```python
from build123d import *

# Parameters (mm, degrees)
CUT_EXTRUDE1_DEPTH  = 153.548755526
CIRPATTERN1_COUNT   = 4
SKETCH6_W           = 0.3175
SKETCH6_H           = 19.05
CUT_EXTRUDE3_DEPTH  = 154.364331947
BOSS_EXTRUDE1_START = 6.19125
SKETCH7_R           = 4.6355
BOSS_EXTRUDE1_DEPTH = 14.76375
FILLET1_R           = 0.9525


with BuildPart() as part:
    # Sketch2 → Revolve1 (revolve)
    with BuildSketch(Plane(origin=(0, 0, 0), x_dir=(0, 0, -1), z_dir=(1, 0, 0)), mode=Mode.PRIVATE) as revolve1_sk:
        Polygon((-133.35, -4.7625), (152.4, -4.7625), (152.4, 0), (-152.4, 0), (-152.4, -4.7625), align=None)
    revolve(revolve1_sk.sketch.rotate(Axis((0, 0, 152.4), (0, 0, -1)), 270), axis=Axis((0, 0, 152.4), (0, 0, -1)))

    # Sketch3 → Cut-Extrude1 (cut, symmetric)
    with BuildSketch(Plane(origin=(0, 0, 0), x_dir=(0, 0, -1), z_dir=(1, 0, 0))):
        Polygon((-152.4, -0.00254), (-133.35, -4.7625), (-152.4, -4.7625), align=None)
    cut_extrude1 = extrude(amount=CUT_EXTRUDE1_DEPTH, both=True, mode=Mode.SUBTRACT)

    # CirPattern1: Cut-Extrude1 ×4 about axis
    cirpattern1_axis = Axis((0, 0, 0), (0, 0, 1))
    for i in range(1, CIRPATTERN1_COUNT):
        add(cut_extrude1.rotate(cirpattern1_axis, i * 360 / CIRPATTERN1_COUNT), mode=Mode.SUBTRACT)

    # Sketch5 → Revolve2 (revolve)
    with BuildSketch(Plane(origin=(0, 0, 0), x_dir=(0, 0, -1), z_dir=(1, 0, 0)), mode=Mode.PRIVATE) as revolve2_sk:
        with BuildLine():
            Line((148.828125, 0), (152.4, 0))
            Line((152.4, 0), (152.4, 8.105021576))
            ThreePointArc((152.4, 8.105021576), (152.243002117, 8.716680214), (151.810824742, 9.177111904))
            ThreePointArc((151.810824742, 9.177111904), (150.6140625, 9.525), (149.417300258, 9.177111904))
            ThreePointArc((149.417300258, 9.177111904), (148.985122883, 8.716680214), (148.828125, 8.105021576))
            Line((148.828125, 8.105021576), (148.828125, 0))
        make_face()
    revolve(revolve2_sk.sketch.rotate(Axis((0, 0, -152.4), (0, 0, 1)), 90), axis=Axis((0, 0, -152.4), (0, 0, 1)))

    # Sketch6 → Cut-Extrude3 (cut, through all)
    with BuildSketch(Plane(origin=(4.7625, 0, 0), x_dir=(0, 0, -1), z_dir=(1, 0, 0))):
        with Locations((140.414375, 0)):
            Rectangle(SKETCH6_W, SKETCH6_H)
        with Locations((142.478125, 0)):
            Rectangle(SKETCH6_W, SKETCH6_H)
        with Locations((141.44625, 0)):
            Rectangle(SKETCH6_W, SKETCH6_H)
        with Locations((139.3825, 0)):
            Rectangle(SKETCH6_W, SKETCH6_H)
        with Locations((138.350625, 0)):
            Rectangle(SKETCH6_W, SKETCH6_H)
        with Locations((137.31875, 0)):
            Rectangle(SKETCH6_W, SKETCH6_H)
        with Locations((136.286875, 0)):
            Rectangle(SKETCH6_W, SKETCH6_H)
        with Locations((135.255, 0)):
            Rectangle(SKETCH6_W, SKETCH6_H)
        with Locations((134.223125, 0)):
            Rectangle(SKETCH6_W, SKETCH6_H)
        with Locations((133.19125, 0)):
            Rectangle(SKETCH6_W, SKETCH6_H)
        with Locations((132.159375, 0)):
            Rectangle(SKETCH6_W, SKETCH6_H)
        with Locations((131.1275, 0)):
            Rectangle(SKETCH6_W, SKETCH6_H)
        with Locations((130.095625, 0)):
            Rectangle(SKETCH6_W, SKETCH6_H)
        with Locations((129.06375, 0)):
            Rectangle(SKETCH6_W, SKETCH6_H)
        with Locations((128.031875, 0)):
            Rectangle(SKETCH6_W, SKETCH6_H)
    extrude(amount=-CUT_EXTRUDE3_DEPTH, mode=Mode.SUBTRACT)


with BuildPart() as cut_extrude3_piece_1:
    # of the separate pieces the step leaves, piece 1, a body of its own (cut_extrude3_pieces)
    add(part.part.solids().sort_by_distance((4.7625, 0, -127.873125))[0])



with BuildPart() as cut_extrude3_piece_2:
    # of the separate pieces the step leaves, piece 2, a body of its own (cut_extrude3_pieces)
    add(part.part.solids().sort_by_distance((-8.105021576, 0, -152.4))[0])


with BuildPart() as cut_extrude3_piece_3:
    # of the separate pieces the step leaves, piece 3, a body of its own (cut_extrude3_pieces)
    add(part.part.solids().sort_by_distance((4.7625, 0, -142.319375))[0])


with BuildPart() as cut_extrude3_piece_4:
    # of the separate pieces the step leaves, piece 4, a body of its own (cut_extrude3_pieces)
    add(part.part.solids().sort_by_distance((4.7625, 0, -141.2875))[0])


with BuildPart() as cut_extrude3_piece_5:
    # of the separate pieces the step leaves, piece 5, a body of its own (cut_extrude3_pieces)
    add(part.part.solids().sort_by_distance((4.7625, 0, -138.191875))[0])


with BuildPart() as cut_extrude3_piece_6:
    # of the separate pieces the step leaves, piece 6, a body of its own (cut_extrude3_pieces)
    add(part.part.solids().sort_by_distance((4.7625, 0, -137.16))[0])


with BuildPart() as cut_extrude3_piece_7:
    # of the separate pieces the step leaves, piece 7, a body of its own (cut_extrude3_pieces)
    add(part.part.solids().sort_by_distance((4.7625, 0, -136.128125))[0])


with BuildPart() as cut_extrude3_piece_8:
    # of the separate pieces the step leaves, piece 8, a body of its own (cut_extrude3_pieces)
    add(part.part.solids().sort_by_distance((4.7625, 0, -134.064375))[0])


with BuildPart() as cut_extrude3_piece_9:
    # of the separate pieces the step leaves, piece 9, a body of its own (cut_extrude3_pieces)
    add(part.part.solids().sort_by_distance((4.7625, 0, -133.0325))[0])


with BuildPart() as cut_extrude3_piece_10:
    # of the separate pieces the step leaves, piece 10, a body of its own (cut_extrude3_pieces)
    add(part.part.solids().sort_by_distance((4.7625, 0, -132.000625))[0])


with BuildPart() as cut_extrude3_piece_11:
    # of the separate pieces the step leaves, piece 11, a body of its own (cut_extrude3_pieces)
    add(part.part.solids().sort_by_distance((4.7625, 0, -130.96875))[0])


with BuildPart() as cut_extrude3_piece_12:
    # of the separate pieces the step leaves, piece 12, a body of its own (cut_extrude3_pieces)
    add(part.part.solids().sort_by_distance((4.7625, 0, -129.936875))[0])


with BuildPart() as cut_extrude3_piece_13:
    # of the separate pieces the step leaves, piece 13, a body of its own (cut_extrude3_pieces)
    add(part.part.solids().sort_by_distance((4.7625, 0, -128.905))[0])


with BuildPart() as cut_extrude3_piece_14:
    # of the separate pieces the step leaves, piece 14, a body of its own (cut_extrude3_pieces)
    add(part.part.solids().sort_by_distance((4.7625, 0, -140.255625))[0])


with BuildPart() as cut_extrude3_piece_15:
    # of the separate pieces the step leaves, piece 15, a body of its own (cut_extrude3_pieces)
    add(part.part.solids().sort_by_distance((4.7625, 0, -139.22375))[0])


with BuildPart() as cut_extrude3_piece_16:
    # of the separate pieces the step leaves, piece 16, a body of its own (cut_extrude3_pieces)
    add(part.part.solids().sort_by_distance((4.7625, 0, -135.09625))[0])


with BuildPart() as cut_extrude3_piece_1_1:
    add(cut_extrude3_piece_1.part)

    add(cut_extrude3_piece_2.part)  # Boss-Extrude1 merges Cut-Extrude3 piece 2

    add(cut_extrude3_piece_3.part)  # Boss-Extrude1 merges Cut-Extrude3 piece 3

    add(cut_extrude3_piece_4.part)  # Boss-Extrude1 merges Cut-Extrude3 piece 4

    add(cut_extrude3_piece_5.part)  # Boss-Extrude1 merges Cut-Extrude3 piece 5

    add(cut_extrude3_piece_6.part)  # Boss-Extrude1 merges Cut-Extrude3 piece 6

    add(cut_extrude3_piece_7.part)  # Boss-Extrude1 merges Cut-Extrude3 piece 7

    add(cut_extrude3_piece_8.part)  # Boss-Extrude1 merges Cut-Extrude3 piece 8

    add(cut_extrude3_piece_9.part)  # Boss-Extrude1 merges Cut-Extrude3 piece 9

    add(cut_extrude3_piece_10.part)  # Boss-Extrude1 merges Cut-Extrude3 piece 10

    add(cut_extrude3_piece_11.part)  # Boss-Extrude1 merges Cut-Extrude3 piece 11

    add(cut_extrude3_piece_12.part)  # Boss-Extrude1 merges Cut-Extrude3 piece 12

    add(cut_extrude3_piece_13.part)  # Boss-Extrude1 merges Cut-Extrude3 piece 13

    add(cut_extrude3_piece_14.part)  # Boss-Extrude1 merges Cut-Extrude3 piece 14

    add(cut_extrude3_piece_15.part)  # Boss-Extrude1 merges Cut-Extrude3 piece 15

    add(cut_extrude3_piece_16.part)  # Boss-Extrude1 merges Cut-Extrude3 piece 16
    # Sketch7 → Boss-Extrude1 (add)
    with BuildSketch(Plane.XY.offset(-148.828125).offset(BOSS_EXTRUDE1_START)):
        with Locations(Location((0, 0, 0), (0, 0, 180))):
            Circle(SKETCH7_R)
    extrude(amount=BOSS_EXTRUDE1_DEPTH)

    # Fillet1
    fillet1_edges = [cut_extrude3_piece_1_1.edges().sort_by_distance(p)[0] for p in [
        (-4.7625, 0, -148.828125),
    ]]
    fillet(fillet1_edges, radius=FILLET1_R)


solid = cut_extrude3_piece_1_1.part
```
The listing builds one solid part. Answer for the finished solid, in the listing's coordinates (mm). A direction names the side the tool comes from. Give positions to 0.01 mm unless a question says otherwise; leave off trailing zeros. Order: outer loops, then holes, each group sorted by start corner. A loop starts at its lowest first (then second) coordinate and runs counter-clockwise, first axis right, second up. Notation, with made-up numbers: M 84.25,-3.5 L 108.25,-3.5 A29 cw 108.25,31.5 Z; hole C -25.5,-9 d8. An arc over 180 degrees is marked long. Put each result on its own line as item: value. Start each with the question number.
Item 1: Which of the six approach directions +Z, -Z, +X, -X, +Y, -Y give full straight-line access (tool end or side, diameter ignored) to faces 1 (the face through (-3.78, 2.9, -140.94)), 2 (the face through (2.88, 0.05, 140.89))?
Item 2: Find the intervals of material crossed by line 1 along Z through (x, y) = (5.5, 2.25); line 2 along X through (y, z) = (1, -39); line 3 along Y through (x, z) = (-0.75, -25), in increasing order.
Item 3: The part is cut by section A-A, the plane z = -52. Determine the outline of the cut face in (x, y) (1 decimal).
Item 4: Flat-ended cylindrical pins translate along their axes: P1, Ø1, axis at x = -1.5, z = 85.5, coming from the +Y side; P2, Ø6, axis at x = 3, z = 91, coming from the -Y side; P3, Ø3, axis at x = 4, z = -83, coming from the +Y side. Find the tip coordinate at first contact, or state that the pin passes through.
Answer key:
1. face 1: +Z
1. face 2: +Z, +X, +Y, -Y
2. line 1: z = -152.4 to -148.83
2. line 2: x = -4.66 to 4.66
2. line 3: y = -4.7 to 4.7
3. outline: C 0,0 d9.5
4. P1: stops at y = 4.66
4. P2: stops at y = -4.76
4. P3: stops at y = 4.05
